```python
from build123d import *

# Parameters (mm, degrees)
SKETCH2_W                = 60
SKETCH2_H                = 60
BOSS_EXTRUDE1_DEPTH      = 89.5
SKETCH3_W                = 56
SKETCH3_H                = 85.5
CUT_EXTRUDE1_DEPTH       = 60
BOSS_EXTRUDE2_DEPTH      = 3
BOSS_EXTRUDE2_DEPTH_BACK = 3
SKETCH4_W                = 3
SKETCH4_H                = 60


with BuildPart() as part:
    # Sketch2 → Boss-Extrude1 (new body)
    with BuildSketch(Plane(origin=(0, 0, 0), x_dir=(1, 0, 0), z_dir=(0, 1, 0))):
        with Locations((-70.647761504, 24.591630357)):
            Rectangle(SKETCH2_W, SKETCH2_H)
    extrude(amount=BOSS_EXTRUDE1_DEPTH)

    # Sketch3 → Cut-Extrude1 (cut)
    with BuildSketch(Plane.XY.offset(5.408369643)):
        with Locations((-70.647761504, 44.75)):
            Rectangle(SKETCH3_W, SKETCH3_H)
    extrude(amount=-CUT_EXTRUDE1_DEPTH, mode=Mode.SUBTRACT)

    # Sketch4 → Boss-Extrude2 (add, two sides: drawn at the far end of the back side and taken through both)
    with BuildSketch(Plane(origin=(0, 89.5, 0), x_dir=(1, 0, 0), z_dir=(0, 1, 0)).offset(-BOSS_EXTRUDE2_DEPTH_BACK)):
        with Locations((-102.147761504, 24.591630357)):
            Rectangle(SKETCH4_W, SKETCH4_H)
        with Locations((-39.147761504, 24.591630357)):
            Rectangle(SKETCH4_W, SKETCH4_H)
    extrude(amount=BOSS_EXTRUDE2_DEPTH + BOSS_EXTRUDE2_DEPTH_BACK)


solid = part.part
```
Source: CAD feature listing. Evaluate the final solid. Frame: model axes, mm. A direction names the side the tool comes from. Give positions to 0.01 mm unless a question says otherwise; leave off trailing zeros. Write each loop counter-clockwise with the first axis right and the second up, starting at its lowest first coordinate (ties: lowest second). Pieces come first, ordered by that corner, then holes.
1. Section query A-A (y = 28). Return the cut outline in (x, z).
2. Section query B-B (x = -51). Return the cut outline in (y, z).
3. Section query C-C (z = -40.5). Return the cut outline in (x, y), then the cut area to 3 significant figures.
4. Material intervals for line 1 along X through (y, z) = (28, -31.5); line 2 along Y through (x, z) = (-49, -18), sorted ascending.
5. Pull-direction query (X, two-part tool) for faces 5 (the face through (-100.648, 43, -24)), 6 (the face through (-37.648, 89, -24)), 7 (the face through (-71, 87.5, -24)), 8 (the face through (-102, 86.5, -25)); classes: +X half, -X half, draft (parallel to the pull), parting line (faces both ways), or undercut.
6. Access query for faces 1 (the face through (-98.648, 44, -24)), 2 (the face through (-40.648, 91, -24)), 3 (the face through (-39, 92.5, -25)), 4 (the face through (-40.648, 43, -24)). Directions: +Z, -Z, +X, -X, +Y, -Y. A direction counts if a zero-diameter tool reaches every point of the face in a straight line with its end or side. Return the directions, or none.
7. First-contact query: pin 1 (12 mm diameter, centred on y = 28.5, z = -27, fed in from +X); pin 2 (18 mm diameter, centred on x = -84.5, z = -30, fed in from +Y); pin 3 (1.5 mm diameter, centred on y = 70, z = -27, fed in from -X); pin 4 (8 mm diameter, centred on x = -93, z = -26, fed in from -Y). Flat tips, straight axial feed; report the tip coordinate or a pass-through.
Output values:
1. outline: (-100.65, -54.59) - (-98.65, -54.59) - (-98.65, 5.41) - (-100.65, 5.41) - close; (-42.65, -54.59) - (-40.65, -54.59) - (-40.65, 5.41) - (-42.65, 5.41) - close
2. outline: (0, -54.59) - (2, -54.59) - (2, 5.41) - (0, 5.41) - close; (87.5, -54.59) - (89.5, -54.59) - (89.5, 5.41) - (87.5, 5.41) - close
3. outline: (-103.65, 86.5) - (-100.65, 86.5) - (-100.65, 0) - (-40.65, 0) - (-40.65, 86.5) - (-37.65, 86.5) - (-37.65, 92.5) - (-40.65, 92.5) - (-40.65, 89.5) - (-100.65, 89.5) - (-100.65, 92.5) - (-103.65, 92.5) - close; hole (-98.65, 2) - (-42.65, 2) - (-42.65, 87.5) - (-98.65, 87.5) - close
3. area: 618 mm2
4. line 1: x = -100.65 to -98.65, -42.65 to -40.65
4. line 2: y = 0 to 2, 87.5 to 89.5
5. face 5: -X half
5. face 6: +X half
5. face 7: undercut
5. face 8: draft
6. face 1: +Z, -Z
6. face 2: +Z, -Z, +Y
6. face 3: +Z, -Z, +X, -X, +Y
6. face 4: +Z, -Z, +X, -Y
7. pin 1: stops at x = -40.65
7. pin 2: stops at y = 89.5
7. pin 3: stops at x = -100.65
7. pin 4: stops at y = 0
